Can you work these out from the drawing? Everything is in mm from the part's minimum corner. A direction names the side the tool comes from. Coordinates: 2 decimals unless noted, no trailing zeros. Loops run counter-clockwise (first coordinate to the right, second up) from the corner with the lowest first, then second, coordinate; pieces in that order, holes last. Notation, with made-up numbers: (56, -11) -> (99, -11) arc R18 ccw to (99, 6) -> close; hole circle Ø4 at (51, 51). An arc over 180 degrees is marked (long way). Put each result on its own line as item: value. Start each with the question number.
Item 1: Will these pins go through, and if not, where does the flat tip stop? P1, Ø1.5, axis at x = 14.5, z = 6.5, coming from the +Y side; P2, Ø1.4, axis at x = 25, y = 14, coming from the +Z side; P3, Ø1.2, axis at x = 27.5, z = 5, coming from the +Y side.
Item 2: For the marked faces 5, 6, 7, 8 and 9, which set-ups out of +Z, -Z, +X, -X, +Y, -Y let a thin tool reach every point of the face, with its end or its side?
Item 3: If we section it at C-C on y = 7.5: Please give me the cut outline in (x, z), plus the area to 3 significant figures.
Item 4: Please list where these lines run through material, in increasing order: L1, parallel to X at y = 7.5, z = 5; L2, parallel to Y at x = 16, z = 3.75; L3, parallel to X at y = 7, z = 5.5. Write a range as from..to.
Item 5: If we section it at B-B on x = 6: Please give me the cut outline in (y, z).
Item 6: We'd pull the mould along X, two halves only. Please class the marked faces 1, 2, 3 and 4: pulls with the +X half, pulls with the -X half, needs draft (parallel to the pull), parting line crosses it, or undercut.
Item 7: If we section it at D-D on z = 8: Please give me the cut outline in (x, y), plus the area to 3 significant figures.
Item 8: If we section it at A-A on z = 5: Please give me the cut outline in (x, y).
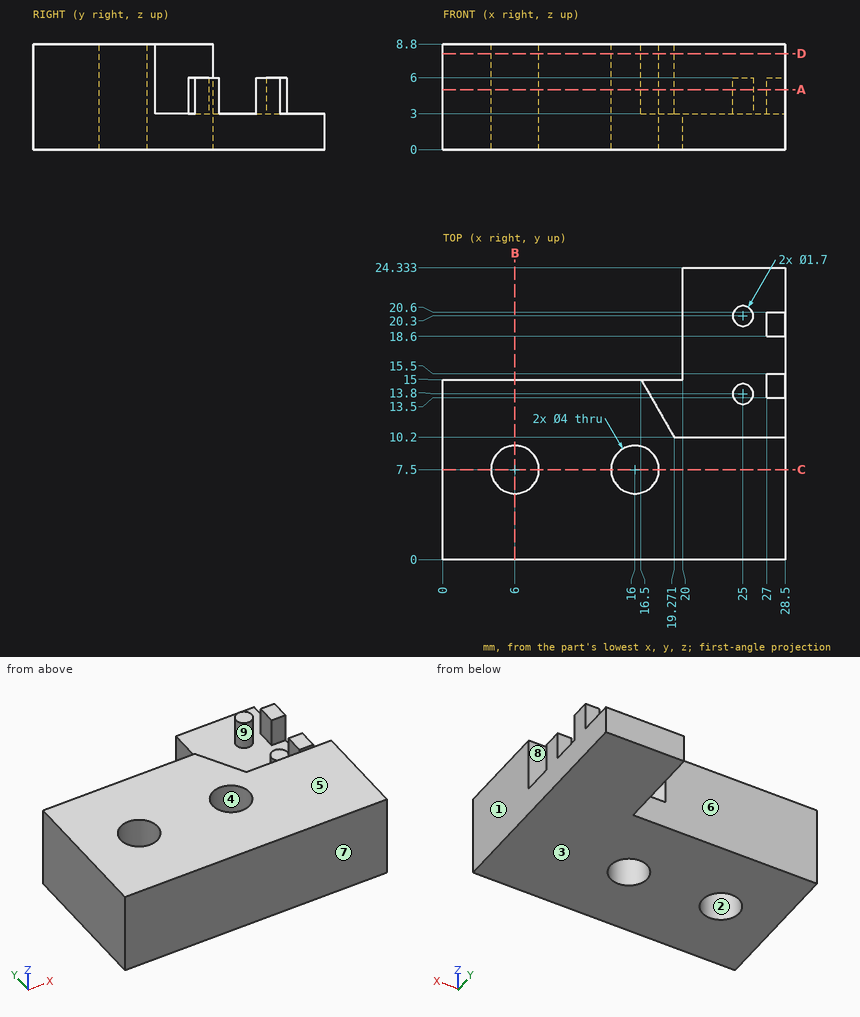
Solutions:
1. P1: y = 15
1. P2: z = 6
1. P3: y = 20.6
2. face 5: +Z, +X, -X, +Y, -Y
2. face 6: +Z, -Z, -X, +Y
2. face 7: +Z, -Z, +X, -X, -Y
2. face 8: +Z, +X
2. face 9: +Z
3. outline: (0, 0) -> (4, 0) -> (4, 8.8) -> (0, 8.8) -> close; (8, 0) -> (14, 0) -> (14, 8.8) -> (8, 8.8) -> close; (18, 0) -> (28.5, 0) -> (28.5, 8.8) -> (18, 8.8) -> close
3. area: 180 mm^2
4. L1: 0..4, 8..14, 18..28.5
4. L2: 0..5.5, 9.5..15
4. L3: 0..4.06, 7.94..14.06, 17.94..28.5
5. outline: (0, 0) -> (5.5, 0) -> (5.5, 8.8) -> (0, 8.8) -> close; (9.5, 0) -> (15, 0) -> (15, 8.8) -> (9.5, 8.8) -> close
6. face 1: pulls with the +X half
6. face 2: undercut
6. face 3: needs draft
6. face 4: undercut
7. outline: (0, 0) -> (28.5, 0) -> (28.5, 10.2) -> (19.27, 10.2) -> (16.5, 15) -> (0, 15) -> close; hole circle Ø4 at (6, 7.5); hole circle Ø4 at (16, 7.5)
7. area: 351 mm^2
8. outline: (0, 0) -> (28.5, 0) -> (28.5, 10.2) -> (19.27, 10.2) -> (16.5, 15) -> (0, 15) -> close; circle Ø1.7 at (25, 13.8); circle Ø1.7 at (25, 20.3); (27, 13.5) -> (28.5, 13.5) -> (28.5, 15.5) -> (27, 15.5) -> close; (27, 18.6) -> (28.5, 18.6) -> (28.5, 20.6) -> (27, 20.6) -> close; hole circle Ø4 at (6, 7.5); hole circle Ø4 at (16, 7.5)
